Autodesk Inventor part; units mm, degrees
ref_plane "YZ Plane" through (0, 0, 0) normal (1, 0, 0) x (0, 1, 0)
ref_plane "XZ Plane" through (0, 0, 0) normal (0, 1, 0) x (-1, 0, 0)
ref_plane "XY Plane" through (0, 0, 0) normal (0, 0, 1) x (1, 0, 0)
sketch "Sketch1" plane through (0, 0, 0) normal (0, 0, 1) x (1, 0, 0)
  line L0 (0, 0) -> (100, 0)
  line L1 (100, 0) -> (100, 65)
  line L2 (100, 65) -> (0, 65)
  line L3 (0, 65) -> (0, 0)
  line L4 (17.5, 48) -> (22.5, 48) construction
  line L5 (17.5, 46.5) -> (22.5, 46.5)
  line L6 (22.5, 49.5) -> (17.5, 49.5)
  arc A0 (17.5, 49.5) -> (17.5, 46.5) centre (17.5, 48) ccw
  arc A1 (22.5, 46.5) -> (22.5, 49.5) centre (22.5, 48) ccw
  line L7 (53.5, 48) -> (48.5, 48) construction
  line L8 (53.5, 49.5) -> (48.5, 49.5)
  line L9 (48.5, 46.5) -> (53.5, 46.5)
  arc A2 (53.5, 46.5) -> (53.5, 49.5) centre (53.5, 48) ccw
  arc A3 (48.5, 49.5) -> (48.5, 46.5) centre (48.5, 48) ccw
  line L10 (17.5, 17) -> (22.5, 17) construction
  line L11 (17.5, 15.5) -> (22.5, 15.5)
  line L12 (22.5, 18.5) -> (17.5, 18.5)
  arc A4 (17.5, 18.5) -> (17.5, 15.5) centre (17.5, 17) ccw
  arc A5 (22.5, 15.5) -> (22.5, 18.5) centre (22.5, 17) ccw
  line L13 (48.5, 17) -> (53.5, 17) construction
  line L14 (48.5, 15.5) -> (53.5, 15.5)
  line L15 (53.5, 18.5) -> (48.5, 18.5)
  arc A6 (48.5, 18.5) -> (48.5, 15.5) centre (48.5, 17) ccw
  arc A7 (53.5, 15.5) -> (53.5, 18.5) centre (53.5, 17) ccw
  line L16 (31.75, 32.5) -> (39.25, 32.5) construction
  line L17 (31.75, 22.5) -> (39.25, 22.5)
  line L18 (39.25, 42.5) -> (31.75, 42.5)
  arc A8 (31.75, 42.5) -> (31.75, 22.5) centre (31.75, 32.5) ccw
  arc A9 (39.25, 22.5) -> (39.25, 42.5) centre (39.25, 32.5) ccw
  circle A10 centre (75, 32.5) radius 11.25
  point P0 (20, 48)
  point P1 (51, 48)
  point P2 (20, 17)
  point P3 (51, 17)
  point P4 (35.5, 32.5)
  point P5 (0, 32.5)
  dimension "d0" = 65
  dimension "d1" = 100
  dimension "d2" = 1.5
  dimension "d3" = 5
  dimension "d4" = 31
  dimension "d5" = 31
  dimension "d6" = 20
  dimension "d7" = 15.5
  dimension "d8" = 15.5
  dimension "d9" = 7.5
  dimension "d10" = 20
  dimension "d11" = 75
  dimension "d12" = 22.5
extrude "Extrusion1" add sketch "Sketch1" along normal blind 6.35
equation "\"d13\" = THICKB"
equation "\"THICKA\" = 3.175"
equation "\"THICKB\" = 6.35"
equation "\"THICKC\" = 12.7"
properties part number "WoodD_Extruder_Side_Motor"
CAD build for the part. Positions are in the model's coordinates, mm. A direction names the side the tool comes from. Give positions to 0.01 mm unless a question says otherwise; leave off trailing zeros. Loops run counter-clockwise (first coordinate to the right, second up) from the corner with the lowest first, then second, coordinate; pieces in that order, holes last. Notation, with made-up numbers: (-25, -36) - (9, -36) arc R30 cw to (9, 3) - close; hole circle Ø7 at (44, 85). An arc over 180 degrees is marked (long way). Put each result on its own line as item: value.
Q1. Probe line 1 along Y through (x, z) = (21, 1.25); line 2 along Y through (x, z) = (75, 3); line 3 along X through (y, z) = (28, 0.75). List the from-to ranges inside material, lowest first.
Filled in:
line 1: y = 0 to 15.5, 18.5 to 46.5, 49.5 to 65
line 2: y = 0 to 21.25, 43.75 to 65
line 3: x = 0 to 22.82, 48.18 to 64.69, 85.31 to 100
Q2. Flat gauge pin, fed straight in: pin 1 (2 mm diameter, centred on x = 47.5, y = 34, fed in from -Z). Where does the tip first touch, or does it go through?
Filled in:
pin 1: passes through
Q3. Mould opens along Y. For faces 1 (the face through (24, 48, 3)), 2 (the face through (51, 15.5, 3)), 3 (the face through (51, 65, 3)), 4 (the face through (49, 26, 6.35)) say: pulls with the +Y half, pulls with the -Y half, needs draft (parallel to the pull), parting line crosses it, or undercut.
Filled in:
face 1: undercut
face 2: undercut
face 3: pulls with the +Y half
face 4: needs draft
Q4. Slice it at A-A (y = 32.5). Give the cut face in (x, z), plus the area to 4 significant figures.
Filled in:
outline: (0, 0) - (21.75, 0) - (21.75, 6.35) - (0, 6.35) - close; (49.25, 0) - (63.75, 0) - (63.75, 6.35) - (49.25, 6.35) - close; (86.25, 0) - (100, 0) - (100, 6.35) - (86.25, 6.35) - close
area: 317.5 mm²
Q5. Slice it at C-C (x = 79). Give the cut face in (y, z).
Filled in:
outline: (0, 0) - (21.99, 0) - (21.99, 6.35) - (0, 6.35) - close; (43.01, 0) - (65, 0) - (65, 6.35) - (43.01, 6.35) - close
Q6. Tool access for faces 5 (the face through (51, 18.5, 3)), 6 (the face through (49, 26, 0)): list every direction of +Z, -Z, +X, -X, +Y, -Y with a clear straight run to the whole face (end or side of a thin tool).
Filled in:
face 5: +Z, -Z
face 6: -Z, +X, -X, +Y, -Y
Q7. Slice it at B-B (z = 3). Give the cut face in (x, y).
Filled in:
outline: (0, 0) - (100, 0) - (100, 65) - (0, 65) - close; hole (17.5, 15.5) - (22.5, 15.5) arc R1.5 ccw to (22.5, 18.5) - (17.5, 18.5) arc R1.5 ccw to start; hole (17.5, 46.5) - (22.5, 46.5) arc R1.5 ccw to (22.5, 49.5) - (17.5, 49.5) arc R1.5 ccw to start; hole (31.75, 22.5) - (39.25, 22.5) arc R10 ccw to (39.25, 42.5) - (31.75, 42.5) arc R10 ccw to start; hole (48.5, 15.5) - (53.5, 15.5) arc R1.5 ccw to (53.5, 18.5) - (48.5, 18.5) arc R1.5 ccw to start; hole (48.5, 46.5) - (53.5, 46.5) arc R1.5 ccw to (53.5, 49.5) - (48.5, 49.5) arc R1.5 ccw to start; hole circle Ø22.5 at (75, 32.5)
Q8. Slice it at D-D (y = 17). Give the cut face in (x, z).
Filled in:
outline: (0, 0) - (16, 0) - (16, 6.35) - (0, 6.35) - close; (24, 0) - (47, 0) - (47, 6.35) - (24, 6.35) - close; (55, 0) - (100, 0) - (100, 6.35) - (55, 6.35) - close
